from build123d import *

# Parameters (mm, degrees)
F0_W     = 76.2
F0_H     = 406.4
F1_DEPTH = 203.2


with BuildPart() as f1:
    # F0 (on Top) → F1 (new body)
    with BuildSketch(Plane.XY):
        Polygon((0, 457.2), (0, 0), (25.4, 0), (101.6, 0), (127, 0), (127, 457.2), (127, 508), (76.2, 508), (76.2, 476.25), (101.6, 476.25), (101.6, 457.2), (76.2, 457.2), (63.5, 457.2), (50.8, 457.2), (25.4, 457.2), (25.4, 476.25), (50.8, 476.25), (50.8, 508), (0, 508), align=None)
        with Locations((63.5, 228.6)):
            Rectangle(F0_W, F0_H, mode=Mode.SUBTRACT)
        Polygon((25.4, 0), (0, 0), (0, -50.8), (50.8, -50.8), (50.8, -19.05), (25.4, -19.05), align=None)
        Polygon((127, 0), (101.6, 0), (101.6, -19.05), (76.2, -19.05), (76.2, -50.8), (127, -50.8), align=None)
    extrude(amount=F1_DEPTH)


solid = f1.part
For this review, take the finished solid that the model builds, in its own axes (mm). A direction names the side the tool comes from. Coordinates: 2 decimals unless noted, no trailing zeros. Order: outer loops, then holes, each group sorted by start corner. A loop starts at its lowest first (then second) coordinate and runs counter-clockwise, first axis right, second up. Notation, with made-up numbers: (-14.75, -12) - (17.25, -12) arc R21 ccw to (17.25, 21) - close; hole circle Ø3 at (19, 18). An arc over 180 degrees is marked (long way). Use one line per item in the form item = value.
Q1. Draft analysis for pull direction X (two halves, no side actions). For faces 6 (the flat face through (25.4, 467, 100)), 7 (the flat face through (101.6, 226, 100)), 8 (the flat face through (25, -50.8, 100)), 9 (the flat face through (0, 233, 100)), state which applies: +X half, -X half, draft (parallel to the pull), parting line (faces both ways), or undercut.
Checked values:
face_6 = undercut
face_7 = undercut
face_8 = draft
face_9 = -X half
Q2. For P1, Ø23, axis at x = 64, z = 95.5, coming from the -Y side, flat-tipped, find the tip position at first contact; note if it passes through.
Checked values:
P1 = 0
Q3. For faces 1 (the flat face through (127, 225, 100)), 2 (the flat face through (64, 457.2, 100)), 3 (the flat face through (50.8, -35, 100)), 4 (the flat face through (50.8, 492, 100)), 5 (the flat face through (101, -50.8, 100)), list the 3-axis set-ups (+Z, -Z, +X, -X, +Y, -Y) from which the entire face can be reached by the end or side of a thin tool; tool diameter is ignored.
Checked values:
face_1 = +Z, -Z, +X, +Y, -Y
face_2 = +Z, -Z
face_3 = +Z, -Z, -Y
face_4 = +Z, -Z, +Y
face_5 = +Z, -Z, +X, -X, -Y
Q4. For probe 1 along Y at (x, z) = (30, 87); probe 2 along X at (y, z) = (32, 47); probe 3 along Y at (x, z) = (66.5, 137), list the stretches that pass through material, from the lowest coordinate up. Write a range as from..to.
Checked values:
probe_1 = -50.8..-19.05, 0..25.4, 431.8..457.2, 476.25..508
probe_2 = 0..25.4, 101.6..127
probe_3 = 0..25.4, 431.8..457.2
Q5. Consider section A-A (y = 248). Give the boundary of the cut face in (x, z), then the cut area to 3 significant figures.
Checked values:
outline = (0, 0) - (25.4, 0) - (25.4, 203.2) - (0, 203.2) - close; (101.6, 0) - (127, 0) - (127, 203.2) - (101.6, 203.2) - close
area = 10,300 mm2
Q6. Consider section B-B (z = 175). Give the boundary of the cut face in (x, y), then the cut area to 3 significant figures.
Checked values:
outline = (0, -50.8) - (50.8, -50.8) - (50.8, -19.05) - (25.4, -19.05) - (25.4, 0) - (101.6, 0) - (101.6, -19.05) - (76.2, -19.05) - (76.2, -50.8) - (127, -50.8) - (127, 508) - (76.2, 508) - (76.2, 476.25) - (101.6, 476.25) - (101.6, 457.2) - (25.4, 457.2) - (25.4, 476.25) - (50.8, 476.25) - (50.8, 508) - (0, 508) - close; hole (25.4, 25.4) - (101.6, 25.4) - (101.6, 431.8) - (25.4, 431.8) - close
area = 35,500 mm2
Q7. Consider section C-C (x = 44.5). Give the boundary of the cut face in (y, z), then the cut area to 3 significant figures.
Checked values:
outline = (-50.8, 0) - (-19.05, 0) - (-19.05, 203.2) - (-50.8, 203.2) - close; (0, 0) - (25.4, 0) - (25.4, 203.2) - (0, 203.2) - close; (431.8, 0) - (457.2, 0) - (457.2, 203.2) - (431.8, 203.2) - close; (476.25, 0) - (508, 0) - (508, 203.2) - (476.25, 203.2) - close
area = 23,200 mm2
